Input: part model. Units: mm. Frame: model coordinates. A direction names the side the tool comes from. Coordinates: 2 decimals unless noted, no trailing zeros. Order: outer loops, then holes, each group sorted by start corner. A loop starts at its lowest first (then second) coordinate and runs counter-clockwise, first axis right, second up. Notation, with made-up numbers: (85.5, 19) - (90.5, 19) arc R13 ccw to (90.5, 28) - close; hole circle Ø4 at (87, 21). An arc over 180 degrees is marked (long way). One line per question, with ' | ' between items. Start each with the question number.
```python
from build123d import *

# Parameters (mm, degrees)
F0_R     = 4
F1_DEPTH = 4
F2_R     = 1
F3_DEPTH = 6
F4_SIZE2 = 2
F4_SIZE  = 0.4
F5_SIZE2 = 2
F5_SIZE  = 2


with BuildPart() as f1:
    # F0 (on Top) → F1 (new body)
    with BuildSketch(Plane.XY):
        Circle(F0_R)
    extrude(amount=F1_DEPTH)

    # F2 (on face) → F3 (join)
    with BuildSketch(Plane.XY.offset(4)):
        Circle(F2_R)
    extrude(amount=F3_DEPTH)

    # F4
    f4_edges = [f1.edges().sort_by_distance(p)[0] for p in [
        (-1, 0, 10),
    ]]
    f4_side = f1.faces().sort_by_distance((0, 0, 10))[0]
    chamfer(f4_edges, length=F4_SIZE, length2=F4_SIZE2, reference=f4_side)

    # F5
    f5_edges = [f1.edges().sort_by_distance(p)[0] for p in [
        (-4, 0, 0),
    ]]
    chamfer(f5_edges, length=F5_SIZE, length2=F5_SIZE2)


solid = f1.part
```
(1) Section D-D (z = 2.25). Output: boundary loops of the cut face in (x, y).
(2) Section A-A (x = 0). Output: boundary loops of the cut face in (y, z).
(3) Section C-C (z = 7.5). Output: boundary loops of the cut face in (x, y).
(4) Pin query (flat end, axial travel): pin 1 (4 mm diameter, centred on x = -2.5, z = 2, fed in from +Y); pin 2 (2 mm diameter, centred on y = 0.5, z = 7, fed in from -X); pin 3 (3 mm diameter, centred on y = 2, z = 6.5, fed in from +X). Return the tip coordinate at first contact, or that it passes through.
(5) Material intervals for line 1 along Z through (x, y) = (-2.5, 1); line 2 along Z through (x, y) = (0.25, 3.25); line 3 along Y through (x, z) = (1.5, 3.75), sorted ascending. Write a range as from..to.
(6) Reachability of faces 1 (the face through (1, -1, 4)), 2 (the face through (0, 0, 10)) from +Z, -Z, +X, -X, +Y, -Y: full face, straight path, thin tool, end or side. Return the list, or none.
Worked answers:
1) outline: circle Ø8 at (0, 0)
2) outline: (-4, 2) - (-2, 0) - (2, 0) - (4, 2) - (4, 4) - (1, 4) - (1, 8) - (0.6, 10) - (-0.6, 10) - (-1, 8) - (-1, 4) - (-4, 4) - close
3) outline: circle Ø2 at (0, 0)
4) pin 1: stops at y = 3.97 | pin 2: stops at x = -1 | pin 3: stops at x = 0.87
5) line 1: z = 0.69..4 | line 2: z = 1.26..4 | line 3: y = -3.71..3.71
6) face 1: +Z | face 2: +Z, +X, -X, +Y, -Y
